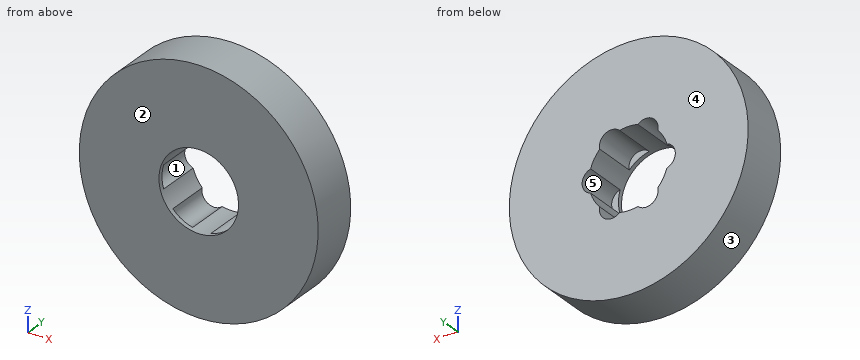
```python
from build123d import *

# Parameters (mm, degrees)
SKETCH1_R           = 45
BOSS_EXTRUDE1_DEPTH = 18
SKETCH2_R           = 15
CUT_EXTRUDE1_DEPTH  = 67.136223055
SKETCH3_R           = 4.526260275
CUT_EXTRUDE2_DEPTH  = 16.327002
CIRPATTERN1_START   = 1.672998056
CIRPATTERN1_DEPTH   = 16.327001944


# Read off the part's stored shape, not the designer's step: CirPattern1
with BuildPart() as part:
    # Sketch1 → Boss-Extrude1 (new body)
    with BuildSketch(Plane(origin=(0, 0, 0), x_dir=(1, 0, 0), z_dir=(0, 1, 0))):
        with Locations(Location((0, 0, 0), (0, 0, 270))):
            Circle(SKETCH1_R)
    extrude(amount=BOSS_EXTRUDE1_DEPTH)

    # Sketch2 → Cut-Extrude1 (cut, through all)
    with BuildSketch(Plane(origin=(0, 0, 0), x_dir=(1, 0, 0), z_dir=(0, 1, 0))):
        with Locations(Location((0, 0, 0), (0, 0, 270))):
            Circle(SKETCH2_R)
    extrude(amount=CUT_EXTRUDE1_DEPTH, mode=Mode.SUBTRACT)

    # Sketch3 → Cut-Extrude2 (cut)
    with BuildSketch(Plane(origin=(0, 18, 0), x_dir=(1, 0, 0), z_dir=(0, 1, 0))):
        with Locations((-13.030483377, 0)):
            Circle(SKETCH3_R)
    extrude(amount=-CUT_EXTRUDE2_DEPTH, mode=Mode.SUBTRACT)

    # CirPattern1 outline → CirPattern1 (cut)
    with BuildSketch(Plane(origin=(0, 0, 0), x_dir=(1, 0, 0), z_dir=(0, 1, 0)).offset(CIRPATTERN1_START)):
        with BuildLine():
            ThreePointArc((-3.435146983, -14.601361759), (-7.5, -12.990381057), (-10.927576721, -10.275605433))
            ThreePointArc((-10.927576721, -10.275605433), (-8.778371826, -15.204586011), (-3.435146983, -14.601361759))
        make_face()
        with BuildLine():
            ThreePointArc((-3.435146983, 14.601361758), (-8.778371826, 15.204586011), (-10.927576721, 10.275605433))
            ThreePointArc((-10.927576721, 10.275605433), (-7.5, 12.990381057), (-3.435146983, 14.601361758))
        make_face()
        with BuildLine():
            ThreePointArc((10.927576721, -10.275605433), (7.5, -12.990381057), (3.435146983, -14.601361759))
            ThreePointArc((3.435146983, -14.601361759), (8.778371826, -15.204586011), (10.927576721, -10.275605433))
        make_face()
        with BuildLine():
            ThreePointArc((10.927576721, 10.275605433), (8.778371826, 15.204586011), (3.435146983, 14.601361758))
            ThreePointArc((3.435146983, 14.601361758), (7.5, 12.990381057), (10.927576721, 10.275605433))
        make_face()
        with BuildLine():
            ThreePointArc((14.362723704, 4.325756326), (15, 0), (14.362723704, -4.325756326))
            ThreePointArc((14.362723704, -4.325756326), (17.556743653, 0), (14.362723704, 4.325756326))
        make_face()
    extrude(amount=CIRPATTERN1_DEPTH, mode=Mode.SUBTRACT)


solid = part.part
```
Could you check a few things on this model? Use its own coordinates, in mm. Face numbers are marked on the shaded views. A direction names the side the tool comes from. Coordinates: 2 decimals unless noted, no trailing zeros. Write each loop counter-clockwise with the first axis right and the second up, starting at its lowest first coordinate (ties: lowest second). Pieces come first, ordered by that corner, then holes. Notation, with made-up numbers: (39.5, 88) - (77.5, 88) arc R20 ccw to (77.5, 117) - close; hole circle Ø2 at (63, 69). An arc over 180 degrees is marked (long way). Use a Markdown table: item, result.
Q1. I'm going to push flat-ended pins straight in: pin 1 Ø2 at (x, y) = (23.5, 4) entering from -Z; pin 2 Ø1.7 at (x, z) = (-7.5, 12.5) entering from +Y; pin 3 Ø3 at (x, y) = (30, 4) entering from +Z; pin 4 Ø18 at (x, z) = (0, 0) entering from +Y. Where does each tip first touch, or does it pass through?
Geometry check:
| item | result |
|---|---|
| pin 1 | stops at z = -38.97 |
| pin 2 | stops at y = 1.67 |
| pin 3 | stops at z = 34.82 |
| pin 4 | passes through |
Q2. Imagine slicing it at D-D (z = -12.5). List the corners of the cut face in (x, y) for me.
Geometry check:
| item | result |
|---|---|
| outline | (-43.23, 0) - (-8.29, 0) - (-8.29, 1.67) - (-10.88, 1.67) - (-10.88, 18) - (-43.23, 18) - close; (8.29, 0) - (43.23, 0) - (43.23, 18) - (10.88, 18) - (10.88, 1.67) - (8.29, 1.67) - close |
Q3. Imagine slicing it at B-B (z = 0). List the corners of the cut face in (x, y) for me, and give its area (3 significant figures).
Geometry check:
| item | result |
|---|---|
| outline | (-45, 0) - (-15, 0) - (-15, 1.67) - (-17.56, 1.67) - (-17.56, 18) - (-45, 18) - close; (15, 0) - (45, 0) - (45, 18) - (17.56, 18) - (17.56, 1.67) - (15, 1.67) - close |
| area | 997 mm2 |
Q4. Which directions (+Z, -Z, +X, -X, +Y, -Y) give clear straight access to the entire face, cutting with the end or side of a thin tool? Please do the marked faces 4 and 5.
Geometry check:
| item | result |
|---|---|
| face 4 | +Z, -Z, +X, -X, +Y |
| face 5 | +Y |
Q5. Imagine slicing it at A-A (x = 0). List the corners of the cut face in (y, z) for me, and give its area (3 significant figures).
Geometry check:
| item | result |
|---|---|
| outline | (0, -45) - (18, -45) - (18, -15) - (0, -15) - close; (0, 15) - (18, 15) - (18, 45) - (0, 45) - close |
| area | 1,080 mm2 |
Q6. Imagine slicing it at C-C (y = 6). List the corners of the cut face in (x, z) for me, and give its area (3 significant figures).
Geometry check:
| item | result |
|---|---|
| outline | circle Ø90 at (0, 0); hole (-14.36, -4.33) arc R15 ccw to (-10.93, -10.28) arc R4.53 ccw to (-3.44, -14.6) arc R15 ccw to (3.44, -14.6) arc R4.53 ccw to (10.93, -10.28) arc R15 ccw to (14.36, -4.33) arc R4.53 ccw to (14.36, 4.33) arc R15 ccw to (10.93, 10.28) arc R4.53 ccw to (3.44, 14.6) arc R15 ccw to (-3.44, 14.6) arc R4.53 ccw to (-10.93, 10.28) arc R15 ccw to (-14.36, 4.33) arc R4.53 ccw to start |
| area | 5,560 mm2 |
Q7. Thinking about a two-plate mould opening in Z: for the marked faces 1, 2 and 3, which applies, +Z half, -Z half, draft (parallel to the pull), parting line (faces both ways), or undercut?
Geometry check:
| item | result |
|---|---|
| face 1 | undercut |
| face 2 | draft |
| face 3 | parting line |
Q8. Please list where these lines run through material, in increasing order: L1, parallel to X at y = 12.5, z = 0; L2, parallel to Z at x = -4, y = 16; L3, parallel to Z at x = 13, y = 2.25.
Geometry check:
| item | result |
|---|---|
| L1 | x = -45 to -17.56, 17.56 to 45 |
| L2 | z = -44.82 to -15.05, 15.05 to 44.82 |
| L3 | z = -43.08 to -7.48, 7.48 to 43.08 |
